```python
from build123d import *

# Parameters (mm, degrees)
ESBO_O2_R                                      = 30
RESSALTO_EXTRUS_O1_DEPTH                       = 20
ESBO_O2_3_R                                    = 30
ESBO_O2_3_R_2                                  = 16
RESSALTO_EXTRUS_O2_DEPTH                       = 25
FILETE1_R                                      = 5
ESBO_O2_4_R                                    = 10
RESSALTO_EXTRUS_O3_DEPTH                       = 120
ESBO_O2_5_R                                    = 10
RESSALTO_EXTRUS_O4_DEPTH                       = 20
BROCA_DE_ROSQUEAR_PARA_TARRAXA_DE_M8X1_2_D     = 6.8
BROCA_DE_ROSQUEAR_PARA_TARRAXA_DE_M8X1_2_DEPTH = 18.127073895
BROCA_DE_ROSQUEAR_PARA_TARRAXA_DE_M8X1_2_TIP   = 2.042926105
BROCA_DE_ROSQUEAR_PARA_TARRAXA_DE_M1_2X0_D     = 6.8
BROCA_DE_ROSQUEAR_PARA_TARRAXA_DE_M1_2X0_DEPTH = 27.957073895
BROCA_DE_ROSQUEAR_PARA_TARRAXA_DE_M1_2X0_TIP   = 2.042926105


with BuildPart() as part:
    # Esboço2 → Ressalto-extrusão1 (new body)
    with BuildSketch(Plane(origin=(0, 0, 0), x_dir=(1, 0, 0), z_dir=(0, 1, 0))):
        with BuildLine():
            ThreePointArc((-142.766795178, -56.646281478), (-143.009054758, -76.280328146), (-127.472672708, -88.287630552))
            ThreePointArc((-127.472672708, -88.287630552), (-118.778190313, -89.570884638), (-110, -90))
            Line((-110, -90), (110, -90))
            ThreePointArc((110, -90), (200, 0), (110, 90))
            Line((110, 90), (-110, 90))
            ThreePointArc((-110, 90), (-117.443432635, 89.691668011), (-124.835864194, 88.76878468))
            ThreePointArc((-124.835864194, 88.76878468), (-140.336700784, 77.939122352), (-141.707084901, 59.079653418))
            ThreePointArc((-141.707084901, 59.079653418), (-146.501498165, 33.18318015), (-171.82521509, 25.94971021))
            ThreePointArc((-171.82521509, 25.94971021), (-191.746461977, 21.825736054), (-199.769091443, 3.130799391))
            ThreePointArc((-199.769091443, 3.130799391), (-192.469638839, -16.620116582), (-171.914884538, -21.189883063))
            ThreePointArc((-171.914884538, -21.189883063), (-145.688040461, -29.338518263), (-142.766795178, -56.646281478))
        make_face()
        with Locations(Location((-110, 0, 0), (0, 0, 270))):
            Circle(ESBO_O2_R, mode=Mode.SUBTRACT)
        with Locations(Location((0, 0, 0), (0, 0, 270))):
            Circle(ESBO_O2_R, mode=Mode.SUBTRACT)
        with Locations(Location((110, 0, 0), (0, 0, 270))):
            Circle(ESBO_O2_R, mode=Mode.SUBTRACT)
    extrude(amount=RESSALTO_EXTRUS_O1_DEPTH)

    # Esboço2<3> → Ressalto-extrusão2 (add)
    # profile 1 of 3: a face of its own
    with BuildSketch(Plane(origin=(0, 0, 0), x_dir=(1, 0, 0), z_dir=(0, 1, 0))):
        with Locations(Location((-110, 0, 0), (0, 0, 270))):
            Circle(ESBO_O2_3_R)
        with Locations(Location((-110, 0, 0), (0, 0, 270))):
            Circle(ESBO_O2_3_R_2, mode=Mode.SUBTRACT)
    # profile 2 of 3: a face of its own
    with BuildSketch(Plane(origin=(0, 0, 0), x_dir=(1, 0, 0), z_dir=(0, 1, 0))):
        with Locations(Location((0, 0, 0), (0, 0, 270))):
            Circle(ESBO_O2_3_R)
        with Locations(Location((0, 0, 0), (0, 0, 270))):
            Circle(ESBO_O2_3_R_2, mode=Mode.SUBTRACT)
    # profile 3 of 3: a face of its own
    with BuildSketch(Plane(origin=(0, 0, 0), x_dir=(1, 0, 0), z_dir=(0, 1, 0))):
        with Locations(Location((110, 0, 0), (0, 0, 270))):
            Circle(ESBO_O2_3_R)
        with Locations(Location((110, 0, 0), (0, 0, 270))):
            Circle(ESBO_O2_3_R_2, mode=Mode.SUBTRACT)
    extrude(amount=RESSALTO_EXTRUS_O2_DEPTH)

    # Filete1
    filete1_edges = [part.edges().sort_by_distance(p)[0] for p in [
        (0, 20, -30),
        (110, 20, -30),
        (-110, 20, -30),
    ]]
    fillet(filete1_edges, radius=FILETE1_R - 0.0001)  # a hair under: the kernel refuses the full size

    # Esboço2<4> → Ressalto-extrusão3 (add)
    with BuildSketch(Plane(origin=(0, 0, 0), x_dir=(1, 0, 0), z_dir=(0, 1, 0))):
        with BuildLine():
            Line((110, 110), (-110, 110))
            ThreePointArc((-110, 110), (-220, 0), (-110, -110))
            Line((-110, -110), (110, -110))
            ThreePointArc((110, -110), (171.017021585, -91.525532377), (211.538461538, -42.307692308))
            ThreePointArc((211.538461538, -42.307692308), (220, 0), (211.538461538, 42.307692308))
            ThreePointArc((211.538461538, 42.307692308), (171.017021585, 91.525532377), (110, 110))
        make_face()
        with Locations(Location((-165, -45.214544805, 0), (0, 0, 270))):
            Circle(ESBO_O2_4_R, mode=Mode.SUBTRACT)
        with Locations(Location((-165, 50, 0), (0, 0, 270))):
            Circle(ESBO_O2_4_R, mode=Mode.SUBTRACT)
        with BuildLine():
            ThreePointArc((-124.835864194, 88.76878468), (-117.443432635, 89.691668011), (-110, 90))
            Line((-110, 90), (110, 90))
            ThreePointArc((110, 90), (200, 0), (110, -90))
            Line((110, -90), (-110, -90))
            ThreePointArc((-110, -90), (-118.778190313, -89.570884638), (-127.472672708, -88.287630552))
            ThreePointArc((-127.472672708, -88.287630552), (-143.009054758, -76.280328146), (-142.766795178, -56.646281478))
            ThreePointArc((-142.766795178, -56.646281478), (-145.688040461, -29.338518263), (-171.914884538, -21.189883063))
            ThreePointArc((-171.914884538, -21.189883063), (-191.224927441, -17.629444698), (-199.999977409, -0.063768613))
            ThreePointArc((-199.999977409, -0.063768613), (-199.945314351, 3.136945366), (-199.776858723, 6.333690699))
            ThreePointArc((-199.776858723, 6.333690699), (-190.469129565, 22.793450693), (-171.82521509, 25.94971021))
            ThreePointArc((-171.82521509, 25.94971021), (-146.501498165, 33.18318015), (-141.707084901, 59.079653418))
            ThreePointArc((-141.707084901, 59.079653418), (-140.336700784, 77.939122352), (-124.835864194, 88.76878468))
        make_face(mode=Mode.SUBTRACT)
    extrude(amount=RESSALTO_EXTRUS_O3_DEPTH)

    # Esboço2<5> → Ressalto-extrusão4 (add)
    with BuildSketch(Plane(origin=(0, 0, 0), x_dir=(1, 0, 0), z_dir=(0, 1, 0))):
        with BuildLine():
            ThreePointArc((230, 30), (218.905996075, 33.358994113), (211.538461538, 42.307692308))
            ThreePointArc((211.538461538, 42.307692308), (220, 0), (211.538461538, -42.307692308))
            ThreePointArc((211.538461538, -42.307692308), (218.905996075, -33.358994113), (230, -30))
            Line((230, -30), (265, -30))
            ThreePointArc((265, -30), (295, 0), (265, 30))
            Line((265, 30), (230, 30))
        make_face()
        with Locations(Location((265, 0, 0), (0, 0, 270))):
            Circle(ESBO_O2_5_R, mode=Mode.SUBTRACT)
    extrude(amount=RESSALTO_EXTRUS_O4_DEPTH)

    # Broca de rosquear para tarraxa de M8x1.253
    with Locations(Plane(origin=(0, 120, 0), x_dir=(1, 0, 0), z_dir=(0, 1, 0))):
        with Locations((-210, 0), (-196.602540378, 50), (-196.602540378, -50), (-110, 100), (-36.666666667, 100), (36.666666667, 100), (110, 100), (177.00903444, 74.227954999), (210, 0), (176.479948314, -77.188918812), (110, -100), (36.666666667, -100), (-36.666666667, -100), (-110, -100)):
            Hole(BROCA_DE_ROSQUEAR_PARA_TARRAXA_DE_M8X1_2_D / 2, depth=BROCA_DE_ROSQUEAR_PARA_TARRAXA_DE_M8X1_2_DEPTH)
            with Locations((0, 0, -(BROCA_DE_ROSQUEAR_PARA_TARRAXA_DE_M8X1_2_DEPTH + BROCA_DE_ROSQUEAR_PARA_TARRAXA_DE_M8X1_2_TIP / 2))):  # 118° drill point
                Cone(0, BROCA_DE_ROSQUEAR_PARA_TARRAXA_DE_M8X1_2_D / 2, BROCA_DE_ROSQUEAR_PARA_TARRAXA_DE_M8X1_2_TIP, mode=Mode.SUBTRACT)

    # Broca de rosquear para tarraxa de M1.2x0.251
    with Locations(Plane(origin=(0, 120, 0), x_dir=(1, 0, 0), z_dir=(0, 1, 0))):
        with Locations((-196.602540378, 50), (-210, 0), (-196.602540378, -50), (-110, -100), (-110, 100), (-36.666666667, 100), (36.666666667, 100), (-36.666666667, -100), (36.666666667, -100), (110, 100), (177.00903444, 74.227954999), (210, 0), (176.479948314, -77.188918812), (110, -100)):
            Hole(BROCA_DE_ROSQUEAR_PARA_TARRAXA_DE_M1_2X0_D / 2, depth=BROCA_DE_ROSQUEAR_PARA_TARRAXA_DE_M1_2X0_DEPTH)
            with Locations((0, 0, -(BROCA_DE_ROSQUEAR_PARA_TARRAXA_DE_M1_2X0_DEPTH + BROCA_DE_ROSQUEAR_PARA_TARRAXA_DE_M1_2X0_TIP / 2))):  # 118° drill point
                Cone(0, BROCA_DE_ROSQUEAR_PARA_TARRAXA_DE_M1_2X0_D / 2, BROCA_DE_ROSQUEAR_PARA_TARRAXA_DE_M1_2X0_TIP, mode=Mode.SUBTRACT)


solid = part.part
```
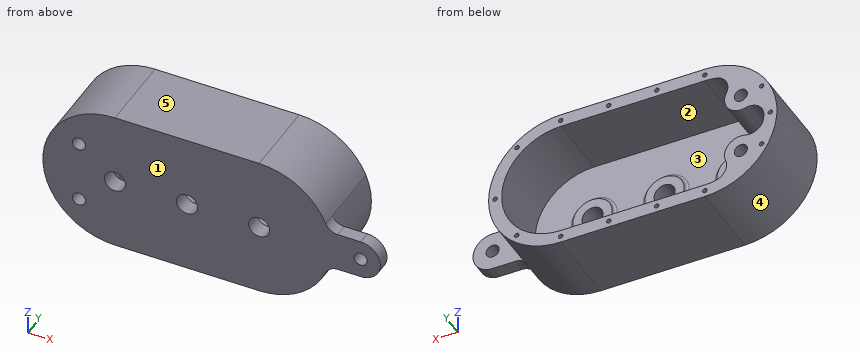
CAD build for the part. Positions are in the model's coordinates, mm. Face numbers are marked on the shaded views. A direction names the side the tool comes from. Round coordinates to 2 decimals unless told otherwise and drop trailing zeros. Write each loop counter-clockwise with the first axis right and the second up, starting at its lowest first coordinate (ties: lowest second). Pieces come first, ordered by that corner, then holes. Notation, with made-up numbers: M 6.5,15 L 19.5,15 A31 cw 19.5,52 Z; hole C 78,-10 d4. An arc over 180 degrees is marked long. One line per question, with ' | ' between items.
1. Cut at C-C on y = 35. Write the cut outline in (x, z), and give its area (3 significant figures).
Working result:
outline: M -110,-110 L 110,-110 A110 ccw 110,110 L -110,110 A110 ccw Z; hole M -200,0.06 A90 ccw -199.78,-6.33 A22 ccw -171.83,-25.95 A25 cw -141.71,-59.08 A22 ccw -124.84,-88.77 A90 ccw -110,-90 L 110,-90 A90 ccw 110,90 L -110,90 A90 ccw -127.47,88.29 A22 ccw -142.77,56.65 A25 cw -171.91,21.19 A22 ccw Z; hole C -165,-50 d20; hole C -165,45.21 d20 | area: 25,200 mm2
2. Which spindle directions (+Z, -Z, +X, -X, +Y, -Y) get a long thin tool onto all of the face, cutting with end or side? Do the marked faces 1 and 2. Say none if no direction does.
Working result:
face 1: +Z, -Z, +X, -X, -Y | face 2: +Y
3. Pin check, flat tips, straight feed: pin 1 Ø3 at (y, z) = (83.5, -44.5) entering from -X; pin 2 Ø4 at (y, z) = (21.5, -51) entering from -X; pin 3 Ø12 at (x, y) = (133, 102) entering from -Z; pin 4 Ø8 at (x, z) = (-110, -100) entering from +Y. Stop position of each tip, or through.
Working result:
pin 1: x = -211.25 | pin 2: x = -208.48 | pin 3: z = -108.68 | pin 4: y = 120
4. Cut at B-B on y = 14.5. Write the cut outline in (x, z).
Working result:
outline: M -110,-110 L 110,-110 A110 ccw 211.54,-42.31 A20 cw 230,-30 L 265,-30 A30 ccw 265,30 L 230,30 A20 cw 211.54,42.31 A110 ccw 110,110 L -110,110 A110 ccw Z; hole M -200,0.06 A90 ccw -199.78,-6.33 A22 cw -199.77,-3.13 A22 cw Z; hole C -165,-50 d20; hole C -165,45.21 d20; hole C -110,0 d32; hole C 0,0 d32; hole C 110,0 d32; hole C 265,0 d20
5. Cut at D-D on y = 108. Count the separate pieces of the cut face and the enclosed holes in it, and give its area (3 significant figures).
Working result:
separate pieces: 1 | enclosed holes: 17 | area: 24,700 mm2
6. Mould opens along X. For the marked faces 3, 4 and 5 say: pulls with the +X half, pulls with the -X half, needs draft (parallel to the pull), parting line crosses it, or undercut.
Working result:
face 3: undercut | face 4: pulls with the -X half | face 5: needs draft
7. Probe L1, parallel to Z at x = 110, y = 108; L2, parallel to Z at x = -10, y = 101; L3, parallel to Z at x = 130.5, y = 24. List the from-to ranges inside material, lowest first. Write a range as from..to.
Working result:
L1: -110..-103.4, -96.6..-90, 90..96.6, 103.4..110 | L2: -110..-90, 90..110 | L3: -108.07..-87.63, -22.04..22.04, 87.63..108.07
